```python
from build123d import *

# Parameters (mm, degrees)
ESQUISSE1_W        = 80
ESQUISSE1_H        = 80
ESQUISSE1_R        = 5
BOSS_EXTRU_1_DEPTH = 5
ESQUISSE2_W        = 10
ESQUISSE2_H        = 5
ESQUISSE2_W_2      = 5
ESQUISSE2_H_2      = 50
CR_NEAUX_DEPTH     = 5


with BuildPart() as part:
    # Esquisse1 → Boss.-Extru.1 (new body)
    with BuildSketch(Plane.XY):
        with Locations((40, 40)):
            Rectangle(ESQUISSE1_W, ESQUISSE1_H)
        with Locations((40, 40)):
            Circle(ESQUISSE1_R, mode=Mode.SUBTRACT)
    extrude(amount=BOSS_EXTRU_1_DEPTH)

    # Esquisse2 → Créneaux - (cut)
    with BuildSketch(Plane.XY.offset(5)):
        with Locations((5, 2.5)):
            Rectangle(ESQUISSE2_W, ESQUISSE2_H)
        with Locations((5, 77.5)):
            Rectangle(ESQUISSE2_W, ESQUISSE2_H)
        with Locations((77.5, 40)):
            Rectangle(ESQUISSE2_W_2, ESQUISSE2_H_2)
        with Locations((72.5, 77.5)):
            Rectangle(ESQUISSE2_W_2, ESQUISSE2_H)
        with Locations((72.5, 2.5)):
            Rectangle(ESQUISSE2_W_2, ESQUISSE2_H)
    extrude(amount=-CR_NEAUX_DEPTH, mode=Mode.SUBTRACT)


solid = part.part
```
Geometry check sheet. Reference: the model listing, model coordinates, mm. A direction names the side the tool comes from. Coordinates: 2 decimals unless noted, no trailing zeros. Write each loop counter-clockwise with the first axis right and the second up, starting at its lowest first coordinate (ties: lowest second). Pieces come first, ordered by that corner, then holes. Notation, with made-up numbers: M 65.25,8 L 94.25,8 A33 ccw 94.25,36 Z; hole C 41,-27 d8. An arc over 180 degrees is marked long. One line per item, written item: value. Start each with the question number.
(1) Sectioned sample at B-B, the plane x = 40. Enter the section's corners in (y, z), and give its area (3 significant figures).
(2) Tool access check on faces 5 (the face through (77, 65, 3)), 6 (the face through (10, 77, 3)), 7 (the face through (72, 75, 3)), 8 (the face through (70, 2, 3)). Record the directions out of +Z, -Z, +X, -X, +Y, -Y that give a thin tool (end or side, any length) a straight path to the whole face; none if there is none.
(3) Sectioned sample at D-D, the plane y = 30. Enter the section's corners in (x, z).
(4) Release check for a two-part mould opening along X. For faces 1 (the face through (75, 2, 3)), 2 (the face through (5, 75, 3)), 3 (the face through (72, 5, 3)), 4 (the face through (80, 7, 2)) record: released by +X, released by -X, zero draft, split by the parting line, or undercut.
(5) Scan lines: line 1 along Y through (x, z) = (40, 3.8); line 2 along X through (y, z) = (60, 1.85); line 3 along Y through (x, z) = (4, 3.65). Record each from-to range of solid material in increasing order. Write a range as [from, to].
(6) Sectioned sample at A-A, the plane z = 0.75. Enter the section's corners in (x, y).
(7) Depth check by flat-ended pin: pin 1 (6 mm diameter, centred on x = 40, y = 40, fed in from -Z); pin 2 (2.5 mm diameter, centred on y = 3, z = 3.5, fed in from -X); pin 3 (1.5 mm diameter, centred on x = 73, z = 2.5, fed in from -Y); pin 4 (2.5 mm diameter, centred on x = 73.5, z = 2, fed in from +Y). Enter the tip coordinate at first touch or a pass-through.
(8) Sectioned sample at C-C, the plane y = 40. Enter the section's corners in (x, z), and give its area (3 significant figures).
Filled sheet:
1. outline: M 0,0 L 35,0 L 35,5 L 0,5 Z; M 45,0 L 80,0 L 80,5 L 45,5 Z
1. area: 350 mm²
2. face 5: +Z, -Z, +X
2. face 6: +Z, -Z, -X, +Y
2. face 7: +Z, -Z, +Y
2. face 8: +Z, -Z, -Y
3. outline: M 0,0 L 75,0 L 75,5 L 0,5 Z
4. face 1: undercut
4. face 2: zero draft
4. face 3: undercut
4. face 4: released by +X
5. line 1: [0, 35], [45, 80]
5. line 2: [0, 75]
5. line 3: [5, 75]
6. outline: M 0,5 L 10,5 L 10,0 L 70,0 L 70,5 L 75,5 L 75,0 L 80,0 L 80,15 L 75,15 L 75,65 L 80,65 L 80,80 L 75,80 L 75,75 L 70,75 L 70,80 L 10,80 L 10,75 L 0,75 Z; hole C 40,40 d10
7. pin 1: through
7. pin 2: x = 10
7. pin 3: y = 5
7. pin 4: y = 75
8. outline: M 0,0 L 35,0 L 35,5 L 0,5 Z; M 45,0 L 75,0 L 75,5 L 45,5 Z
8. area: 325 mm²
